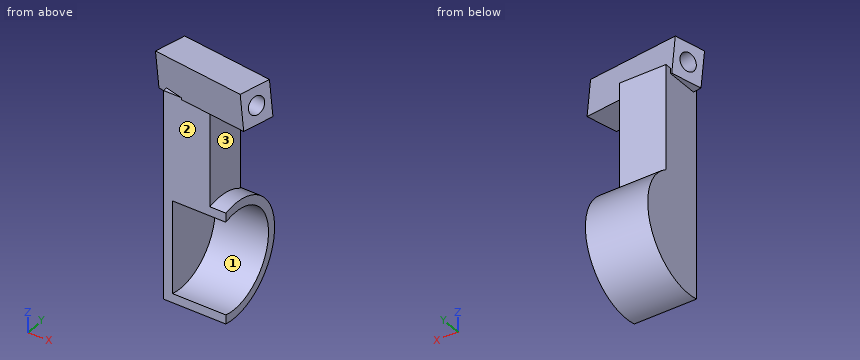
from build123d import *

# Parameters (mm, degrees)
EXTRUDE_1_DEPTH      = 35
SKETCH_6_W           = 60
SKETCH_6_H           = 25
EXTRUDE_2_DEPTH      = 26
SKETCH_4_R           = 27.5
CUT_EXTRUDE_1_DEPTH  = 30
EXTRUDE_3_DEPTH      = 22
EXTRUDE_3_DEPTH_BACK = 38
SKETCH_12_W          = 20
SKETCH_12_H          = 18
SKETCH_12_R          = 5


with BuildPart() as part:
    # Sketch 2 → Extrude 1 (new body)
    with BuildSketch(Plane(origin=(0, 0, 0), x_dir=(0, 0, -1), z_dir=(1, 0, 0))):
        with BuildLine():
            Line((-31.622776602, -7.5), (31.622776602, -7.5))
            ThreePointArc((31.622776602, -7.5), (0, 32.5), (-31.622776602, -7.5))
        make_face()
    extrude(amount=EXTRUDE_1_DEPTH)

    # Sketch 6 → Extrude 2 (add)
    with BuildSketch(Plane.ZY):
        with Locations((57.386127875, 5)):
            Rectangle(SKETCH_6_W, SKETCH_6_H)
    extrude(amount=-EXTRUDE_2_DEPTH)

    # Sketch 4 → Cut-Extrude 1 (cut)
    with BuildSketch(Plane(origin=(35, 0, 0), x_dir=(0, 0, -1), z_dir=(1, 0, 0))):
        Circle(SKETCH_4_R)
    extrude(amount=-CUT_EXTRUDE_1_DEPTH, mode=Mode.SUBTRACT)

    # Sketch 12 → Extrude 3 (add, two sides: drawn at the far end of the back side and taken through both)
    with BuildSketch(Plane(origin=(17, 0, 97), x_dir=(-0.12015591727422713, 0.0308332759507369, 0.9922761030268414), z_dir=(-0.9611356730519813, 0.246637553152495, -0.12404892325959627)).offset(-EXTRUDE_3_DEPTH_BACK)):
        Rectangle(SKETCH_12_W, SKETCH_12_H)
        with Locations(Location((0, 0, 0), (0, 0, 270))):
            Circle(SKETCH_12_R, mode=Mode.SUBTRACT)
    extrude(amount=EXTRUDE_3_DEPTH + EXTRUDE_3_DEPTH_BACK)


solid = part.part
Part model, mm, in its own coordinate system. Face numbers are marked on the shaded views. Round coordinates to 2 decimals unless told otherwise and drop trailing zeros. Write each loop counter-clockwise with the first axis right and the second up, starting at its lowest first coordinate (ties: lowest second). Pieces come first, ordered by that corner, then holes. Notation, with made-up numbers: M 58,53.5 L 96,53.5 A27 ccw 96,82.5 Z; hole C 58.25,89.25 d3. An arc over 180 degrees is marked long. Return JSON: item names as keys, results as strings. Group by question number.
(1) Saw through at B-B on z = 0. Write the cut outline in (x, y), then the cut area to 3 significant figures.
(2) Drill centre lines: probe 1 along Z at (x, y) = (15, 0); probe 2 along Z at (x, y) = (24, 0); probe 3 along Y at (x, z) = (11.5, 0). Where is each one in solid material? Low to high.
(3) Pin check, flat tips, straight feed: pin 1 Ø6 at (y, z) = (25, 8.5) entering from -X; pin 2 Ø1 at (x, z) = (20.5, -15) entering from +Y; pin 3 Ø13 at (x, z) = (18.5, 71) entering from +Y. Stop position of each tip, or through.
(4) Saw through at D-D on z = 36. Write the cut outline in (x, y).
(5) Saw through at A-A on y = 26. Write the cut outline in (x, z), then the cut area to 3 significant figures.
(6) Saw through at C-C on x = 33. Count the separate pieces of the cut face and the enclosed holes in it, then the cut area to 3 significant figures.
(7) Two-plate mould, pull along Z, no slides. Class the marked faces 1, 2 and 3: +Z half, -Z half, draft (parallel to the pull), parting line (faces both ways), or undercut.
Returned:
{
 "1": {"outline": "M 0,-7.5 L 5,-7.5 L 5,27.5 L 35,27.5 L 35,32.5 L 0,32.5 Z", "area": "350 mm²"},
 "2": {"probe 1": "-32.5 to -27.5, 27.5 to 91.74, 101.77 to 106.84", "probe 2": "-32.5 to -27.5, 27.5 to 87.39, 87.77 to 93.12, 102.57 to 107.93", "probe 3": "27.5 to 32.5"},
 "3": {"pin 1": "x = 0", "pin 2": "y = 29.09", "pin 3": "y = 17.5"},
 "4": {"outline": "M 0,-7.5 L 26,-7.5 L 26,17.5 L 0,17.5 Z"},
 "5": {"outline": "M 0,-19.5 L 35,-19.5 L 35,-8.96 L 5,-8.96 L 5,8.96 L 35,8.96 L 35,19.5 L 0,19.5 Z", "area": "828 mm²"},
 "6": {"separate pieces": "2", "enclosed holes": "1", "area": "840 mm²"},
 "7": {"face 1": "undercut", "face 2": "draft", "face 3": "undercut"}
}
